Design review of the part built by this model. Coordinates are the model's own, in mm. Round coordinates to 2 decimals unless told otherwise and drop trailing zeros. Loops run counter-clockwise (first coordinate to the right, second up) from the corner with the lowest first, then second, coordinate; pieces in that order, holes last. Notation, with made-up numbers: (78, -32) -> (116, -32) arc R34 cw to (116, 6) -> close; hole circle Ø9 at (1, 26). An arc over 180 degrees is marked (long way). Answer as CSV lines item,"result". Start each with the question number.
```python
from build123d import *

# Parameters (mm, degrees)
BOSS_EXTRUDE1_DEPTH = 2
SKETCH8_W           = 25.4
SKETCH8_H           = 25.4
BOSS_EXTRUDE2_DEPTH = 2


with BuildPart() as part:
    # Sketch1 → Boss-Extrude1 (new body)
    with BuildSketch(Plane(origin=(0, 0, 0), x_dir=(1, 0, 0), z_dir=(0, 1, 0))):
        Polygon((-29.123295379, 223.557352941), (8.976704621, 223.557352941), (8.976704621, 20.357352941), (-5.310795379, 20.357352941), (-5.310795379, -5.042647059), (-14.835795379, -5.042647059), (-14.835795379, 20.357352941), (-29.123295379, 20.357352941), align=None)
    extrude(amount=BOSS_EXTRUDE1_DEPTH)

    # Sketch8 → Boss-Extrude2 (add)
    with BuildSketch(Plane(origin=(0, 2, 0), x_dir=(1, 0, 0), z_dir=(0, 1, 0))):
        with Locations((-27.535795379, 7.657352941)):
            Rectangle(SKETCH8_W, SKETCH8_H)
        with Locations((7.389204621, 7.657352941)):
            Rectangle(SKETCH8_W, SKETCH8_H)
    extrude(amount=-BOSS_EXTRUDE2_DEPTH)


solid = part.part
```
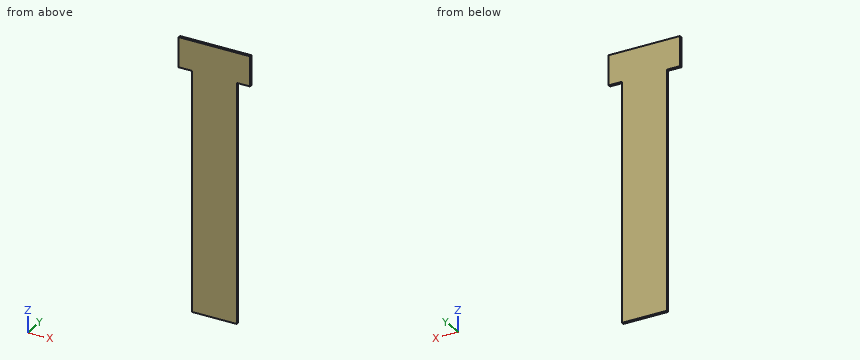
Q1. For pin 1 Ø1 at (x, y) = (15.5, 1.5) entering from -Z; pin 2 Ø1 at (y, z) = (0.5, -34.5) entering from +X, all flat-tipped, find the tip position at first contact; note any pin that passes through.
Q2. To check wall thickness, follow probe 1 along X at (y, z) = (1.6, -63.5); probe 2 along Z at (x, y) = (-37.5, 1.9). State the ranges of each line that lie inside material, in increasing order. Write a range as from..to.
Q3. Add section C-C, the plane x = -36. Give the boundary of the cut face in (y, z).
Q4. Add section A-A, the plane y = 1.6. Give the boundary of the cut face in (x, z).
Q5. Add section B-B, the plane z = -29. Give the boundary of the cut face in (x, y), and give its area (3 significant figures).
Worked answers:
1,pin 1,"stops at z = -20.36"
1,pin 2,"stops at x = 8.98"
2,probe 1,"x = -29.12..8.98"
2,probe 2,"z = -20.36..5.04"
3,outline,"(0, -20.36) -> (2, -20.36) -> (2, 5.04) -> (0, 5.04) -> close"
4,outline,"(-40.24, -20.36) -> (-29.12, -20.36) -> (-29.12, -223.56) -> (8.98, -223.56) -> (8.98, -20.36) -> (20.09, -20.36) -> (20.09, 5.04) -> (-40.24, 5.04) -> close"
5,outline,"(-29.12, 0) -> (8.98, 0) -> (8.98, 2) -> (-29.12, 2) -> close"
5,area,"76.2 mm^2"
